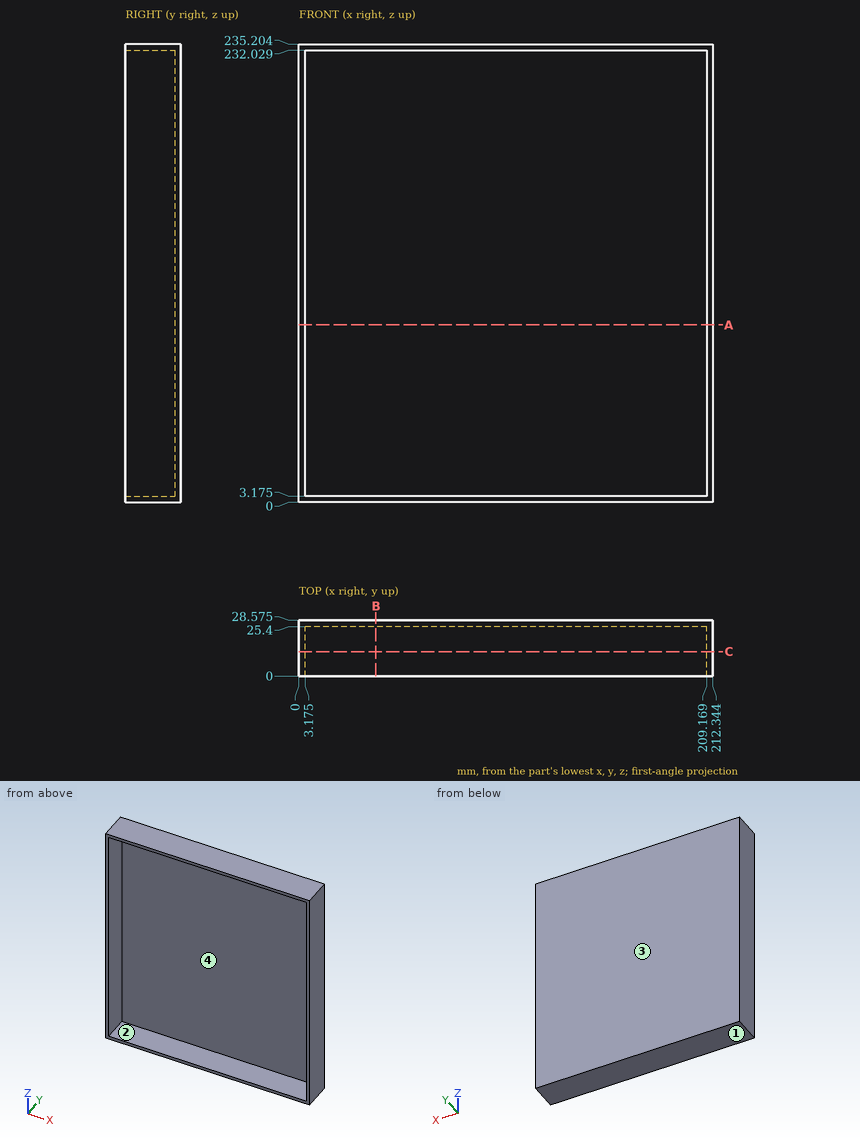
Here's the drawing with two shaded views (mm, measured from the low corner). I have some questions. A direction names the side the tool comes from. Coordinates: 2 decimals unless noted, no trailing zeros. Write each loop counter-clockwise with the first axis right and the second up, starting at its lowest first coordinate (ties: lowest second). Pieces come first, ordered by that corner, then holes. Notation, with made-up numbers: M -35.5,22 L 2.5,22 A18 ccw 2.5,50 Z; hole C 80.25,66.5 d2. An arc over 180 degrees is marked long. Write item = value, one per line. Start each with the question number.
Q1. If we section it at B-B, the plane x = 39.5: Write out the boundary of the cut face in (y, z) (3 decimals), then the cut area to 3 significant figures.
Q2. If we section it at A-A, the plane z = 91: Write out the boundary of the cut face in (x, y) (3 decimals), then the cut area to 3 significant figures.
Q3. If I drill on L1, parallel to X at y = 5, z = 72 (3 decimals); L2, parallel to Z at x = 138, y = 11.5 (3 decimals); L3, parallel to Y at x = 189, z = 205.5 (3 decimals), over which ranges is the centre line in solid material (lowest first)? Write a range as [from, to].
Q4. I'm going to push flat-ended pins straight in: pin 1 (8 mm diameter, centred on x = 104, z = 59, fed in from -Y); pin 2 (4 mm diameter, centred on x = 46.5, y = 22, fed in from -Z). Where does each tip first touch, or does it pass through?
Q5. On a 3-axis mill with a long thin cutter (end or side, diameter ignored), from which of +Z, -Z, +X, -X, +Y, -Y can I reach the whole of each face in a straight line? I mean the marked faces 3 and 4. Say none if no direction works.
Q6. Thinking about a two-plate mould opening in X: for the marked faces 1 and 2, which applies, released by +X, released by -X, zero draft, split by the parting line, or undercut?
Q7. If we section it at C-C, the plane y = 12.5: Write out the boundary of the cut face in (x, z) (3 decimals), then the cut area to 3 significant figures.
Check sheet entries:
q1.outline = M 0,0 L 28.575,0 L 28.575,235.204 L 0,235.204 L 0,232.029 L 25.4,232.029 L 25.4,3.175 L 0,3.175 Z
q1.area = 908 mm²
q2.outline = M 0,0 L 3.175,0 L 3.175,25.4 L 209.169,25.4 L 209.169,0 L 212.344,0 L 212.344,28.575 L 0,28.575 Z
q2.area = 835 mm²
q3.L1 = [0, 3.175], [209.169, 212.344]
q3.L2 = [0, 3.175], [232.029, 235.204]
q3.L3 = [25.4, 28.575]
q4.pin_1 = 25.4
q4.pin_2 = 0
q5.face_3 = +Z, -Z, +X, -X, +Y
q5.face_4 = -Y
q6.face_1 = zero draft
q6.face_2 = undercut
q7.outline = M 0,0 L 212.344,0 L 212.344,235.204 L 0,235.204 Z; hole M 3.175,3.175 L 209.169,3.175 L 209.169,232.029 L 3.175,232.029 Z
q7.area = 2,800 mm²
